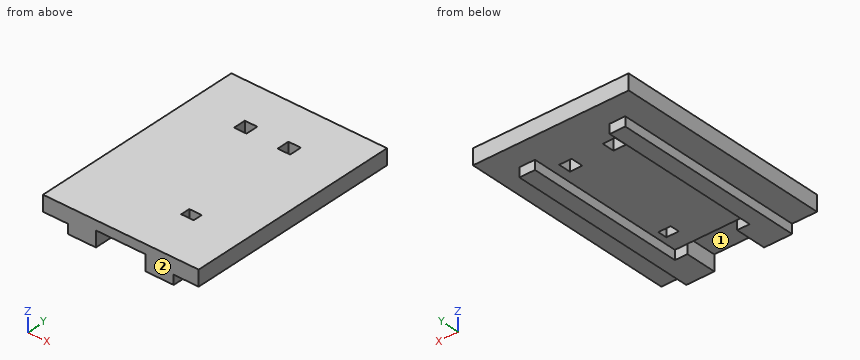
Autodesk Inventor part; units mm, degrees
ref_plane "YZ Plane" through (0, 0, 0) normal (1, 0, 0) x (0, 1, 0)
ref_plane "XZ Plane" through (0, 0, 0) normal (0, 1, 0) x (-1, 0, 0)
ref_plane "XY Plane" through (0, 0, 0) normal (0, 0, 1) x (1, 0, 0)
sketch "Sketch1" plane through (0, 0, 0) normal (0, 0, 1) x (1, 0, 0)
  line L0 (0, 0) -> (17, 0)
  line L1 (17, 0) -> (17, 31)
  line L2 (17, 31) -> (0, 31)
  line L3 (0, 31) -> (0, 0)
  dimension "d0" = 17
  dimension "d1" = 31
extrude "Extrusion1" add sketch "Sketch1" along normal blind 1.5
sketch "Sketch2" plane through (0, 0, 1.5) normal (0, 0, 1) x (1, 0, 0)
  line L0 (17, 31) -> (0, 31)
  line L1 (2.5, 31) -> (14.5, 31)
  line L2 (14.5, 31) -> (14.5, 5)
  line L3 (14.5, 5) -> (2.5, 5)
  line L4 (2.5, 5) -> (2.5, 31)
  line L5 (0, 0) -> (17, 0)
  line L6 (4.5, 0) -> (12.5, 0)
  line L7 (12.5, 0) -> (12.5, 5)
  line L8 (12.5, 5) -> (4.5, 5)
  line L9 (4.5, 5) -> (4.5, 0)
  line L10 (0, 31) -> (0, 0)
  point P0 (4.5, 5)
  dimension "d4" = 12
  dimension "d5" = 8
  dimension "d6" = 5
  dimension "d7" = 17
  dimension "d8" = 2.5
  dimension "d9" = 4.5
extrude "Extrusion2" cut sketch "Sketch2" against normal up to surface (1.5 mm away) contours L2 L3 L4 L0 | L7 L5 L9 L3
sketch "Sketch3" plane through (0, 0, 1.5) normal (0, 0, 1) x (1, 0, 0)
  line L0 (-4, 35) -> (21, 35)
  line L1 (21, 35) -> (21, 0)
  line L2 (21, 0) -> (-4, 0)
  line L3 (-4, 0) -> (-4, 35)
  line L4 (2.5, 31) -> (0, 31)
  line L5 (0, 31) -> (0, 0)
  line L6 (17, 0) -> (17, 31)
  line L7 (0, 0) -> (4.5, 0)
  dimension "d12" = 4
  dimension "d13" = 4
  dimension "d14" = 4
extrude "Extrusion3" add sketch "Sketch3" along normal blind 2.5
sketch "Sketch4" plane through (0, 0, 1.5) normal (0, 0, -1) x (-1, 0, 0)
  line L0 (0, 0) -> (-4.5, 0)
  line L1 (-4.5, 0) -> (-12.5, 0)
  line L2 (-12.5, 0) -> (-12.5, 5)
  line L3 (-12.5, 5) -> (-4.5, 5)
  line L4 (-4.5, 5) -> (-4.5, 0)
extrude "Extrusion4" cut sketch "Sketch4" against normal blind 1
sketch "Sketch5" plane through (0, 0, 1.5) normal (0, 0, -1) x (-1, 0, 0)
  line L0 (-11.5, 7.75) -> (-13.5, 7.75)
  line L1 (-13.5, 7.75) -> (-13.5, 9.25)
  line L2 (-13.5, 9.25) -> (-11.5, 9.25)
  line L3 (-11.5, 9.25) -> (-11.5, 7.75)
  line L4 (-12.5, 5) -> (-4.5, 5)
  line L5 (-4.5, 5) -> (-4.5, 0)
  line L6 (-12.5, 0) -> (-12.5, 5)
  point P0 (0, 0)
  dimension "d19" = 2
  dimension "d20" = 1.5
  dimension "d21" = 2.75
  dimension "d25" = 1
extrude "Extrusion5" cut sketch "Sketch5" against normal through all
sketch "Sketch6" plane through (0, 0, 1.5) normal (0, 0, -1) x (-1, 0, 0)
  line L0 (-4, 26.25) -> (-6, 26.25)
  line L1 (-6, 26.25) -> (-6, 28.25)
  line L2 (-6, 28.25) -> (-4, 28.25)
  line L3 (-4, 28.25) -> (-4, 26.25)
  line L4 (-2.5, 31) -> (0, 31)
  line L5 (-2.5, 5) -> (-2.5, 31)
  line L6 (0, 31) -> (0, 0)
  line L7 (-12.5, 5) -> (-4.5, 5)
  line L8 (-8.5, 5) -> (-8.5, 35)
  line L9 (-21, 35) -> (4, 35)
  line L10 (-13, 26.25) -> (-11, 26.25)
  line L11 (-11, 26.25) -> (-11, 28.25)
  line L12 (-11, 28.25) -> (-13, 28.25)
  line L13 (-13, 28.25) -> (-13, 26.25)
  dimension "d26" = 2.75
  dimension "d27" = 2
  dimension "d28" = 2
  dimension "d30" = 4
extrude "Extrusion6" cut sketch "Sketch6" against normal through all
equation "\"d8\" = -0.5 * d4 + 0.5 * d7"
equation "\"d9\" = -0.5 * d5 + 0.5 * d7"
properties part number "ds input capture cover v1"
Could you check a few things on this model? Use its own coordinates, in mm. Face numbers are marked on the shaded views. Round coordinates to 2 decimals unless told otherwise and drop trailing zeros. Order: outer loops, then holes, each group sorted by start corner. A loop starts at its lowest first (then second) coordinate and runs counter-clockwise, first axis right, second up.
(1) Please list where these lines run through material, in increasing order: line 1 along X through (y, z) = (26.5, 3.2); line 2 along Y through (x, z) = (5.5, 1.75); line 3 along Y through (x, z) = (12.25, 3.3).
Response values:
line 1: x = -4 to 4, 6 to 11, 13 to 21
line 2: y = 5 to 26.25, 28.25 to 35
line 3: y = 0 to 7.75, 9.25 to 26.25, 28.25 to 35
(2) Imagine slicing it at A-A (z = 0.45). Write out the boundary of the cut face in (x, y), plus the area to 3 significant figures.
Response values:
outline: (0, 0) - (4.5, 0) - (4.5, 5) - (2.5, 5) - (2.5, 31) - (0, 31) - close; (12.5, 0) - (17, 0) - (17, 31) - (14.5, 31) - (14.5, 5) - (12.5, 5) - close
area: 175 mm2
(3) I'm going to push flat-ended pins straight in: pin 1 (2.5 mm diameter, centred on x = 9.5, y = 3, fed in from -Z); pin 2 (1.2 mm diameter, centred on y = 8.5, z = 0.5, fed in from -X); pin 3 (1.6 mm diameter, centred on y = 15.5, z = 0.5, fed in from +X). Where does each tip first touch, or does it pass through?
Response values:
pin 1: stops at z = 2.5
pin 2: stops at x = 0
pin 3: stops at x = 17
(4) Imagine slicing it at B-B (x = 8.5). Write out the boundary of the cut face in (y, z), plus the area to 3 significant figures.
Response values:
outline: (0, 2.5) - (5, 2.5) - (5, 1.5) - (35, 1.5) - (35, 4) - (0, 4) - close
area: 82.5 mm2
(5) Imagine slicing it at C-C (z = 2.1). Write out the boundary of the cut face in (x, y).
Response values:
outline: (-4, 0) - (4.5, 0) - (4.5, 5) - (12.5, 5) - (12.5, 0) - (21, 0) - (21, 35) - (-4, 35) - close; hole (4, 26.25) - (6, 26.25) - (6, 28.25) - (4, 28.25) - close; hole (11, 26.25) - (13, 26.25) - (13, 28.25) - (11, 28.25) - close; hole (11.5, 7.75) - (13.5, 7.75) - (13.5, 9.25) - (11.5, 9.25) - close
(6) If we mould it in two halves opening along X, with no side actions, what happens to the marked faces 1 and 2? For each: released by +X, released by -X, zero draft, split by the parting line, or undercut.
Response values:
face 1: undercut
face 2: zero draft
(7) Imagine slicing it at D-D (y = 14.5). Write out the boundary of the cut face in (x, z), plus the area to 3 significant figures.
Response values:
outline: (-4, 1.5) - (0, 1.5) - (0, 0) - (2.5, 0) - (2.5, 1.5) - (14.5, 1.5) - (14.5, 0) - (17, 0) - (17, 1.5) - (21, 1.5) - (21, 4) - (-4, 4) - close
area: 70.0 mm2
